Can you work these out from the model? Positions are in its coordinate system, mm. Coordinates: 2 decimals unless noted, no trailing zeros. Order: outer loops, then holes, each group sorted by start corner. A loop starts at its lowest first (then second) coordinate and runs counter-clockwise, first axis right, second up. Notation, with made-up numbers: (87, 17) -> (118, 17) arc R34 cw to (118, 52) -> close; hole circle Ø10 at (12.25, 36.5). An arc over 180 degrees is marked (long way). Return JSON: item names as keys, results as strings. Group by question number.
1) If we section it at A-A, the plane y = 4: Please give me the cut outline in (x, z).
2) If we section it at C-C, the plane z = 1.75: Please give me the cut outline in (x, y) (3 decimals).
3) If we section it at D-D, the plane x = -25: Please give me the cut outline in (y, z), then the cut area to 4 significant figures.
4) If we section it at B-B, the plane x = 6: Please give me the cut outline in (y, z) (3 decimals).
5) For pin 1 (4 mm diameter, centred on x = 6, y = 0, fed in from -Z), with a flat end and sliding along its axis, tell me the tip position at first contact or that it passes through.
6) If I drill on probe 1 along Y at (x, z) = (-18, 2.8); probe 2 along X at (y, z) = (-2, 1.6); probe 3 along Y at (x, z) = (6, 0.55) (3 decimals), over which ranges is the centre line in solid material (lowest first)? Write a range as from..to.
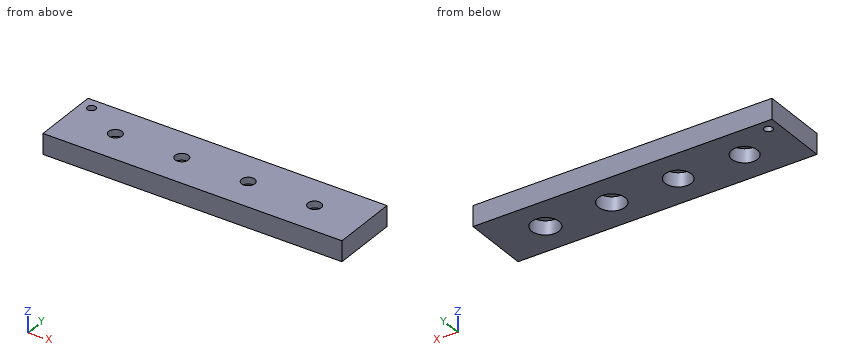
from build123d import *

# Parameters (mm, degrees)
COUPON_BAR_54X12X3P7_PROFILE_W                 = 54
COUPON_BAR_54X12X3P7_PROFILE_H                 = 12
COUPON_BAR_54X12X3P7_DEPTH                     = 3.7
PRESS_SOCKETS_4P65_4P75_4P85_4P95_DE_2_R       = 2.325
PRESS_SOCKETS_4P65_4P75_4P85_4P95_DE_2_R_2     = 2.375
PRESS_SOCKETS_4P65_4P75_4P85_4P95_DE_2_R_3     = 2.425
PRESS_SOCKETS_4P65_4P75_4P85_4P95_DE_2_R_4     = 2.475
PRESS_SOCKETS_4P65_4P75_4P85_4P95_DEPTH2_DEPTH = 2.5
M2_CENTRE_SCREW_CLEARANCE_START                = -50
M2_CENTRE_SCREW_CLEARANCE_PROFILE_R            = 1.2
M2_CENTRE_SCREW_CLEARANCE_DEPTH                = 78.90501747
ORIENTATION_MARK_AT_SMALLEST_SOCKET_START      = -50
ORIENTATION_MARK_AT_SMALLEST_SOCKET_PROF_R     = 0.75
ORIENTATION_MARK_AT_SMALLEST_SOCKET_DEPTH      = 78.90501747


with BuildPart() as part:
    # Coupon_bar_54x12x3p7_profile → Coupon_bar_54x12x3p7 (new body)
    with BuildSketch(Plane.XY):
        Rectangle(COUPON_BAR_54X12X3P7_PROFILE_W, COUPON_BAR_54X12X3P7_PROFILE_H)
    extrude(amount=COUPON_BAR_54X12X3P7_DEPTH)

    # Press_sockets_4p65_4p75_4p85_4p95_de 2 → Press_sockets_4p65_4p75_4p85_4p95_depth2 (cut)
    with BuildSketch(Plane.XY):
        with Locations((-18, 0)):
            Circle(PRESS_SOCKETS_4P65_4P75_4P85_4P95_DE_2_R)
        with Locations((-6, 0)):
            Circle(PRESS_SOCKETS_4P65_4P75_4P85_4P95_DE_2_R_2)
        with Locations((6, 0)):
            Circle(PRESS_SOCKETS_4P65_4P75_4P85_4P95_DE_2_R_3)
        with Locations((18, 0)):
            Circle(PRESS_SOCKETS_4P65_4P75_4P85_4P95_DE_2_R_4)
    extrude(amount=PRESS_SOCKETS_4P65_4P75_4P85_4P95_DEPTH2_DEPTH, mode=Mode.SUBTRACT)

    # M2_centre_screw_clearance_profile → M2_centre_screw_clearance (cut, through all)
    with BuildSketch(Plane.XY.offset(M2_CENTRE_SCREW_CLEARANCE_START)):
        with Locations(Location((-18, 0, 0), (0, 0, 180))):
            Circle(M2_CENTRE_SCREW_CLEARANCE_PROFILE_R)
        with Locations(Location((-6, 0, 0), (0, 0, 180))):
            Circle(M2_CENTRE_SCREW_CLEARANCE_PROFILE_R)
        with Locations(Location((6, 0, 0), (0, 0, 180))):
            Circle(M2_CENTRE_SCREW_CLEARANCE_PROFILE_R)
        with Locations(Location((18, 0, 0), (0, 0, 180))):
            Circle(M2_CENTRE_SCREW_CLEARANCE_PROFILE_R)
    extrude(amount=M2_CENTRE_SCREW_CLEARANCE_DEPTH, mode=Mode.SUBTRACT)

    # Orientation_mark_at_smallest_socket_profile → Orientation_mark_at_smallest_socket (cut, through all)
    with BuildSketch(Plane.XY.offset(ORIENTATION_MARK_AT_SMALLEST_SOCKET_START)):
        with Locations(Location((-25, 4, 0), (0, 0, 180))):
            Circle(ORIENTATION_MARK_AT_SMALLEST_SOCKET_PROF_R)
    extrude(amount=ORIENTATION_MARK_AT_SMALLEST_SOCKET_DEPTH, mode=Mode.SUBTRACT)


solid = part.part
Result sheet:
{
 "1": {"outline": "(-27, 0) -> (-25.75, 0) -> (-25.75, 3.7) -> (-27, 3.7) -> close; (-24.25, 0) -> (27, 0) -> (27, 3.7) -> (-24.25, 3.7) -> close"},
 "2": {"outline": "(-27, -6) -> (27, -6) -> (27, 6) -> (-27, 6) -> close; hole circle Ø1.5 at (-25, 4); hole circle Ø4.65 at (-18, 0); hole circle Ø4.75 at (-6, 0); hole circle Ø4.85 at (6, 0); hole circle Ø4.95 at (18, 0)"},
 "3": {"outline": "(-6, 0) -> (3.25, 0) -> (3.25, 3.7) -> (-6, 3.7) -> close; (4.75, 0) -> (6, 0) -> (6, 3.7) -> (4.75, 3.7) -> close", "area": "38.85 mm2"},
 "4": {"outline": "(-6, 0) -> (-2.425, 0) -> (-2.425, 2.5) -> (-1.2, 2.5) -> (-1.2, 3.7) -> (-6, 3.7) -> close; (1.2, 2.5) -> (2.425, 2.5) -> (2.425, 0) -> (6, 0) -> (6, 3.7) -> (1.2, 3.7) -> close"},
 "5": {"pin 1": "stops at z = 2.5"},
 "6": {"probe 1": "y = -6..-1.2, 1.2..6", "probe 2": "x = -27..-19.19, -16.81..-7.28, -4.72..4.63, 7.37..16.54, 19.46..27", "probe 3": "y = -6..-2.425, 2.425..6"}
}
